```python
from build123d import *

# Parameters (mm, degrees)
F0_R     = 5
F1_DEPTH = 12
F3_R     = 5
F4_DEPTH = 0.6


with BuildPart() as f1:
    # F0 (on Right) → F1 (new body)
    with BuildSketch(Plane.YZ):
        Circle(F0_R)
        with BuildLine():
            ThreePointArc((1.5, 2), (0, -2.5), (-1.5, 2))
            Line((-1.5, 2), (1.5, 2))
        make_face(mode=Mode.SUBTRACT)
    extrude(amount=F1_DEPTH)

    # F3 (on face) → F4 (join)
    with BuildSketch(Plane(origin=(0, 0, 0), x_dir=(0, -1, 0), z_dir=(-1, 0, 0))):
        Circle(F3_R)
    extrude(amount=-F4_DEPTH)

    # F2 (on Top) → F5 (revolve)
    with BuildSketch(Plane.XY):
        with BuildLine():
            Line((0, 0.498465), (0, 5))
            Line((0, 5), (-2, 7))
            ThreePointArc((-2, 7), (-0.544714, 3.889288), (0, 0.498465))
        make_face()
    revolve(axis=Axis((-3.519394, 0, 0), (-1, 0, 0)))


solid = f1.part
```
Geometry check sheet. Reference: the model listing, model coordinates, mm. Round coordinates to 2 decimals unless told otherwise and drop trailing zeros. Order: outer loops, then holes, each group sorted by start corner. A loop starts at its lowest first (then second) coordinate and runs counter-clockwise, first axis right, second up. Notation, with made-up numbers: M 80.5,-12.5 L 118.5,-12.5 A19 ccw 118.5,9.5 Z; hole C -2.75,18.25 d9. An arc over 180 degrees is marked long. Write item = value, one per line.
Q1. Scan lines: line 1 (Z direction, x = 6.25, y = 0); line 2 (Z direction, x = 3.5, y = 1.5); line 3 (Y direction, x = 8.75, z = 1). Record each from-to range of solid material in increasing order.
Answer block:
line_1 = -5 to -2.5, 2 to 5
line_2 = -4.77 to -2, 2 to 4.77
line_3 = -4.9 to -2.29, 2.29 to 4.9
Q2. Depth check by flat-ended pin: pin 1 Ø4 at (y, z) = (0, 0) entering from -X; pin 2 Ø8 at (x, z) = (10, 1.5) entering from -Y; pin 3 Ø0.9 at (x, y) = (7.5, 0.5) entering from -Z. Enter the tip coordinate at first touch or a pass-through.
Answer block:
pin_1 = -0.12
pin_2 = -5
pin_3 = -5
Q3. Release check for a two-part mould opening along Z. For faces 1 (the cylindrical face through (5.92, -1.08, -4.88)), 2 (the flat face through (6, 0, 2)), 3 (the flat face through (0, 0, 0)), 4 (the flat face through (12, -0.1, 2.3)) record: released by +Z, released by -Z, zero draft, split by the parting line, or undercut.
Answer block:
face_1 = split by the parting line
face_2 = undercut
face_3 = undercut
face_4 = zero draft
Q4. Section check A-A (x = 9.25). Enter the section's corners in (y, z), plus the area to 3 significant figures.
Answer block:
outline = C 0,0 d10; hole M -1.5,2 A2.5 ccw long 1.5,2 Z
area = 59.9 mm^2
